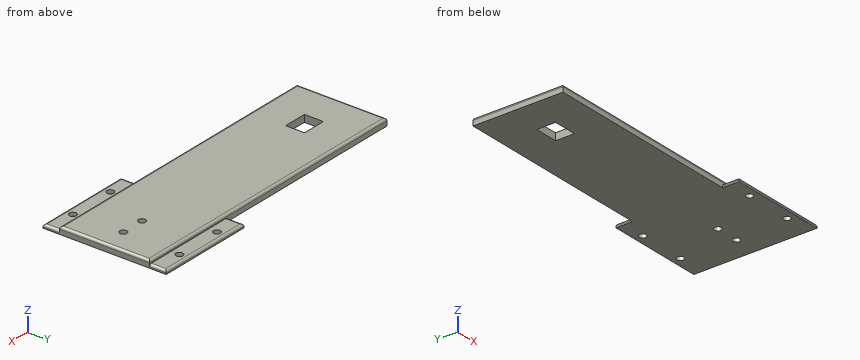
Autodesk Inventor part; units mm, degrees
ref_plane "YZ Plane" through (0, 0, 0) normal (1, 0, 0) x (0, 1, 0)
ref_plane "XZ Plane" through (0, 0, 0) normal (0, 1, 0) x (-1, 0, 0)
ref_plane "XY Plane" through (0, 0, 0) normal (0, 0, 1) x (1, 0, 0)
sketch "sketch" plane through (0, 0, 0) normal (0, 0, 1) x (1, 0, 0)
  line L0 (-52.714, 0) -> (218.2838, 0) construction
  line L1 (0, -17.4) -> (0, 55.4) construction
  line L2 (0, 38) -> (126.5, 38)
  line L3 (126.5, 38) -> (126.5, 0)
  line L4 (126.5, 0) -> (0, 0)
  line L5 (0, 0) -> (0, 38)
  line L6 (15, 23) -> (25, 23)
  line L7 (25, 23) -> (25, 15)
  line L8 (25, 15) -> (15, 15)
  line L9 (15, 15) -> (15, 23)
  circle A0 centre (116.5, 19) radius 1.5
  circle A1 centre (106.5, 19) radius 1.5
  line L10 (85, 45) -> (126.5, 45)
  line L11 (126.5, 45) -> (126.5, 38)
  line L12 (126.5, 38) -> (85, 38)
  line L13 (85, 38) -> (85, 45)
  line L14 (-14, 19) -> (179.5698, 19) construction
  circle A2 centre (95, 41.5) radius 1.5
  circle A3 centre (115, 41.5) radius 1.5
  line L15 (85, -7) -> (126.5, -7)
  line L16 (126.5, -7) -> (126.5, 0)
  line L17 (85, 0) -> (85, -7)
  circle A4 centre (95, -3.5) radius 1.5
  circle A5 centre (115, -3.5) radius 1.5
  dimension "d0" = 126.5
  dimension "d1" = 38
  dimension "d2" = 15
  dimension "d3" = 10
  dimension "d4" = 8
  dimension "d5" = 15
  dimension "d6" = 3
  dimension "d7" = 10
  dimension "d8" = 3
  dimension "d9" = 10
  dimension "d10" = 19
  dimension "d11" = 19
  dimension "d12" = 41.5
  dimension "d13" = 7
  dimension "d14" = 19
  dimension "d15" = 10
  dimension "d16" = 11.5
  dimension "d17" = 3
  dimension "d18" = 3
  dimension "d19" = 3.5
  dimension "d20" = 3.5
extrude "roof" add sketch "sketch" along normal blind 3 contours L2 L3 L4 L5
extrude "bolt" add sketch "sketch" along normal blind 1.5 contours L13 L10 L11 L2 | L4 L16 L15 L17
fillet "so_hurt" radius 1 10 edges at (63.25, 38, 3) (63.25, 0, 3) (126.5, 19, 3) (85, -3.5, 1.5) (105.75, -7, 1.5) (126.5, 41.5, 1.5) (105.75, 45, 1.5) (85, 41.5, 1.5) (0, 19, 3) (126.5, -3.5, 1.5)
equation "\"d8\" = d6"
equation "\"d10\" = 0.5 * d1"
equation "\"d11\" = 0.5 * d1"
equation "\"d14\" = 0.5 * d1"
equation "\"d17\" = d6"
equation "\"d18\" = d6"
equation "\"d19\" = 0.5 * d13"
equation "\"d20\" = 0.5 * d13"
properties part number "roof"
Work out the finished part from the listing and answer in its coordinate system (mm). Give positions to 0.01 mm unless a question says otherwise; leave off trailing zeros. Order: outer loops, then holes, each group sorted by start corner. A loop starts at its lowest first (then second) coordinate and runs counter-clockwise, first axis right, second up. Notation, with made-up numbers: (35.5, -16) - (47.5, -16) arc R9 cw to (47.5, -9) - close; hole circle Ø7 at (59.5, -19). An arc over 180 degrees is marked (long way). One line per item, written item: value. Start each with the question number.
1. Consider line 1 (Y direction, x = 95, z = 0.4); line 2 (Y direction, x = 95, z = 0.95); line 3 (Y direction, x = 17.5, z = 0.95). Determine where each line is inside the solid, lowest interval first.
2. Each of these flat-tipped pins is pushed along its axis until it touches: pin 1 Ø1.8 at (x, y) = (108.5, 40) entering from +Z; pin 2 Ø1.8 at (x, y) = (95, 41.5) entering from -Z; pin 3 Ø0.6 at (x, z) = (77.5, 0.5) entering from -Y. Where does it stop, or does it pass through?
3. Section C-C, the plane x = 30 is taken. Write down the section's boundary in (y, z), then the cut area to 3 significant figures.
4. Section A-A, the plane x = 95 is taken. Write down the section's boundary in (y, z), then the cut area to 3 significant figures.
5. Section B-B, the plane y = 41.5 is taken. Write down the section's boundary in (x, z), then the cut area to 3 significant figures.
Filled sheet:
1. line 1: -7 to -5, -2 to 40, 43 to 45
1. line 2: -6.89 to -5, -2 to 40, 43 to 44.89
1. line 3: 0 to 15, 23 to 38
2. pin 1: z = 1.5
2. pin 2: through
2. pin 3: y = 0
3. outline: (0, 0) - (38, 0) - (38, 2) arc R1 ccw to (37, 3) - (1, 3) arc R1 ccw to (0, 2) - close
3. area: 114 mm²
4. outline: (-7, 0) - (-5, 0) - (-5, 1.5) - (-6, 1.5) arc R1 ccw to (-7, 0.5) - close; (-2, 0) - (40, 0) - (40, 1.5) - (38, 1.5) - (38, 2) arc R1 ccw to (37, 3) - (1, 3) arc R1 ccw to (0, 2) - (0, 1.5) - (-2, 1.5) - close; (43, 0) - (45, 0) - (45, 0.5) arc R1 ccw to (44, 1.5) - (43, 1.5) - close
4. area: 125 mm²
5. outline: (85, 0) - (93.5, 0) - (93.5, 1.5) - (86, 1.5) arc R1 ccw to (85, 0.5) - close; (96.5, 0) - (113.5, 0) - (113.5, 1.5) - (96.5, 1.5) - close; (116.5, 0) - (126.5, 0) - (126.5, 0.5) arc R1 ccw to (125.5, 1.5) - (116.5, 1.5) - close
5. area: 52.8 mm²
